```python
from build123d import *

# Parameters (mm, degrees)
SKETCH_1_W      = 70
SKETCH_1_H      = 74
SKETCH_1_R      = 1.5
EXTRUDE_1_DEPTH = 1.5
EXTRUDE_2_DEPTH = 16
SKETCH_3_W      = 7.90187143
SKETCH_3_H      = 34.179510185
SKETCH_3_W_2    = 8.610784302
SKETCH_3_W_3    = 7.635032944
SKETCH_3_H_2    = 12.090105775
EXTRUDE_3_DEPTH = 8
SKETCH_4_W      = 48.879724418
SKETCH_4_H      = 46.217704607
EXTRUDE_4_DEPTH = 1.5


with BuildPart() as part:
    # 草图1 → 凸台-拉伸1 (new body)
    with BuildSketch(Plane(origin=(0, 0, 0), x_dir=(1, 0, 0), z_dir=(0, 1, 0))):
        Rectangle(SKETCH_1_W, SKETCH_1_H)
        with Locations(Location((4, 22, 0), (0, 0, 270))):
            Circle(SKETCH_1_R, mode=Mode.SUBTRACT)
        with Locations(Location((-12, 2, 0), (0, 0, 270))):
            Circle(SKETCH_1_R, mode=Mode.SUBTRACT)
        with Locations(Location((20, 2, 0), (0, 0, 270))):
            Circle(SKETCH_1_R, mode=Mode.SUBTRACT)
        with Locations(Location((4, -18, 0), (0, 0, 270))):
            Circle(SKETCH_1_R, mode=Mode.SUBTRACT)
    extrude(amount=EXTRUDE_1_DEPTH)

    # 草图2 → 凸台-拉伸2 (add)
    with BuildSketch(Plane(origin=(0, 1.5, 0), x_dir=(1, 0, 0), z_dir=(0, 1, 0))):
        with BuildLine():
            Line((-35, 35.5), (-28, 35.5))
            ThreePointArc((-28, 35.5), (-25.878679656, 34.621320344), (-25, 32.5))
            Line((-25, 32.5), (-25, -4.5))
            ThreePointArc((-25, -4.5), (-25.878679656, -6.621320344), (-28, -7.5))
            Line((-28, -7.5), (-35, -7.5))
            ThreePointArc((-35, -7.5), (-35.707106781, -7.207106781), (-36, -6.5))
            Line((-36, -6.5), (-36, 34.5))
            ThreePointArc((-36, 34.5), (-35.707106781, 35.207106781), (-35, 35.5))
        make_face()
    extrude(amount=EXTRUDE_2_DEPTH)

    # 草图3 → 凸台-拉伸3 (add)
    with BuildSketch(Plane(origin=(0, 1.5, 0), x_dir=(1, 0, 0), z_dir=(0, 1, 0))):
        with Locations((-18.962737702, 12.563109243)):
            Rectangle(SKETCH_3_W, SKETCH_3_H)
        with Locations((29.139365584, 12.563109243)):
            Rectangle(SKETCH_3_W_2, SKETCH_3_H)
        with Locations((28.656584238, -26.076525333)):
            Rectangle(SKETCH_3_W_3, SKETCH_3_H_2)
    extrude(amount=EXTRUDE_3_DEPTH)

    # 草图4 → 凸台-拉伸4 (add)
    with BuildSketch(Plane(origin=(0, 9.5, 0), x_dir=(1, 0, 0), z_dir=(0, 1, 0))):
        with Locations((5.477124507, 11.306310679)):
            Rectangle(SKETCH_4_W, SKETCH_4_H)
    extrude(amount=EXTRUDE_4_DEPTH)


solid = part.part
```
The model under review builds one solid part; all positions refer to its coordinate system, in mm. A direction names the side the tool comes from. Round coordinates to 2 decimals unless told otherwise and drop trailing zeros. Write each loop counter-clockwise with the first axis right and the second up, starting at its lowest first coordinate (ties: lowest second). Pieces come first, ordered by that corner, then holes.
(1) We need section A-A on z = -2. Give the boundary of the cut face in (x, y), and give its area (3 significant figures).
(2) Insertion check: pin 1 (4.5 mm diameter, centred on x = -20, z = -12, fed in from +Y); pin 2 (8 mm diameter, centred on y = 9, z = -7, fed in from +X); pin 3 (8.5 mm diameter, centred on x = 29, z = 26, fed in from +Y). Each pin has a flat end and moves straight along its axis. Give the tip position at first contact, or say it passes through.
(3) We need section D-D on x = 20. Give the boundary of the cut face in (y, z).
(4) We need section C-C on y = 6. Give the boundary of the cut face in (x, z).
(5) We need section B-B on x = -1.5. Give the boundary of the cut face in (y, z), and give its area (3 significant figures).
(6) Mouldability with a two-part tool opening along Z and no side actions: class faces 1 (the flat face through (29, 5, -29.653)), 2 (the flat face through (5, 11, -12)), 3 (the cylindrical face through (4.07, 0.74, -23.5)) as +Z half, -Z half, draft (parallel to the pull), parting line (faces both ways), or undercut.
(7) Wall thickness on L1, parallel to X at y = 1.05, z = -2; L2, parallel to Z at x = 30, y = 2.5; L3, parallel to X at y = 0.95, z = 18: over which ranges is each line inside the solid? List them lowest first.
(8) Machinability: for faces 4 (the flat face through (-22.914, 5, -12)), 5 (the flat face through (32, 9.5, -13)), 6 (the flat face through (-19, 5, -29.653)), 7 (the flat face through (29, 5, 32.122)), which of the approach directions +Z, -Z, +X, -X, +Y, -Y give a long, thin tool a straight path to every point of the face, cutting with its end or side? Answer none if there is none.
Findings below:
1. outline: (-36, 1.5) - (-35, 1.5) - (-35, 0) - (-13.5, 0) - (-13.5, 1.5) - (-15.01, 1.5) - (-15.01, 9.5) - (24.83, 9.5) - (24.83, 1.5) - (21.5, 1.5) - (21.5, 0) - (35, 0) - (35, 1.5) - (33.44, 1.5) - (33.44, 9.5) - (29.92, 9.5) - (29.92, 11) - (-18.96, 11) - (-18.96, 9.5) - (-22.91, 9.5) - (-22.91, 1.5) - (-25, 1.5) - (-25, 17.5) - (-36, 17.5) - close; (-10.5, 0) - (18.5, 0) - (18.5, 1.5) - (-10.5, 1.5) - close
1. area: 477 mm2
2. pin 1: stops at y = 11
2. pin 2: stops at x = 33.44
2. pin 3: stops at y = 9.5
3. outline: (0, -37) - (1.5, -37) - (1.5, -3.5) - (0, -3.5) - close; (0, -0.5) - (1.5, -0.5) - (1.5, 37) - (0, 37) - close; (9.5, -34.42) - (11, -34.42) - (11, 11.8) - (9.5, 11.8) - close
4. outline: (-36, -34.5) arc R1 ccw to (-35, -35.5) - (-28, -35.5) arc R3 ccw to (-25, -32.5) - (-25, 4.5) arc R3 ccw to (-28, 7.5) - (-35, 7.5) arc R1 ccw to (-36, 6.5) - close; (-22.91, -29.65) - (-15.01, -29.65) - (-15.01, 4.53) - (-22.91, 4.53) - close; (24.83, -29.65) - (33.44, -29.65) - (33.44, 4.53) - (24.83, 4.53) - close; (24.84, 20.03) - (32.47, 20.03) - (32.47, 32.12) - (24.84, 32.12) - close
5. outline: (0, -37) - (1.5, -37) - (1.5, 37) - (0, 37) - close; (9.5, -34.42) - (11, -34.42) - (11, 11.8) - (9.5, 11.8) - close
5. area: 180 mm2
6. face 1: -Z half
6. face 2: draft
6. face 3: undercut
7. L1: x = -35 to -13.5, -10.5 to 18.5, 21.5 to 35
7. L2: z = -29.65 to 4.53, 20.03 to 32.12
7. L3: x = -35 to 2.5, 5.5 to 35
8. face 4: +Z, -Z, +Y
8. face 5: +Z, -Z, +X, +Y
8. face 6: -Z, +X
8. face 7: +Z, +X, -X, +Y
